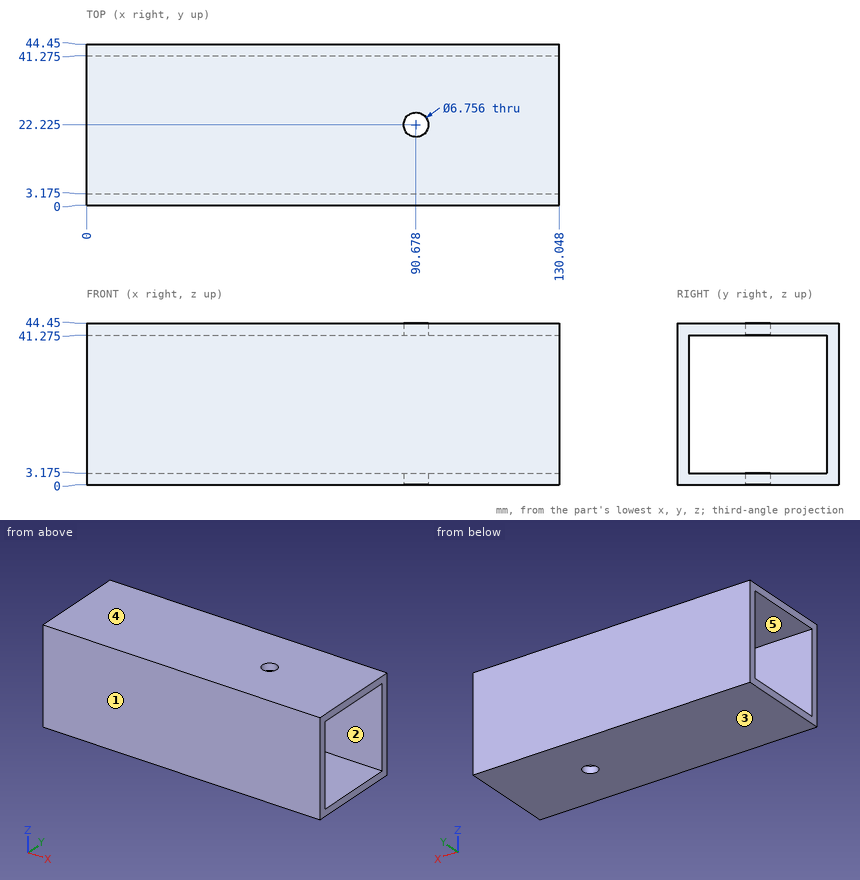
Can you work these out from the drawing? Everything is in mm from the part's minimum corner. A direction names the side the tool comes from. Round coordinates to 2 decimals unless told otherwise and drop trailing zeros.
1. For the marked faces 4 and 5, which set-ups out of +Z, -Z, +X, -X, +Y, -Y let a thin tool reach every point of the face, with its end or its side?
2. If we mould it in two halves opening along Y, with no side actions, what happens to the marked faces 1, 2 and 3? For each: released by +Y, released by -Y, zero draft, split by the parting line, or undercut.
3. Will this pin go through, and if not, where does the flat tip stop? pin 1 Ø5.5 at (x, y) = (90.678, 22.225) entering from +Z.
Answer sheet:
1. face 4: +Z, +X, -X, +Y, -Y
1. face 5: +X, -X
2. face 1: released by -Y
2. face 2: undercut
2. face 3: zero draft
3. pin 1: passes through
